Source: CAD feature listing. Evaluate the final solid. Frame: model axes, mm. A direction names the side the tool comes from. Give positions to 0.01 mm unless a question says otherwise; leave off trailing zeros. Write each loop counter-clockwise with the first axis right and the second up, starting at its lowest first coordinate (ties: lowest second). Pieces come first, ordered by that corner, then holes. Notation, with made-up numbers: M -4,37 L 5,37 A32 ccw 5,75 Z; hole C -7,-35.5 d3. An arc over 180 degrees is marked long. Return JSON: item names as keys, results as strings.
```python
from build123d import *

# Parameters (mm, degrees)
SKETCH_2_W          = 6.5
SKETCH_2_H          = 35
EXTRUDE_1_DEPTH     = 5
SKETCH_3_W          = 2.5
SKETCH_3_H          = 2
CUT_EXTRUDE_1_DEPTH = 180
SKETCH_4_W          = 6.5
SKETCH_4_H          = 19
EXTRUDE_2_DEPTH     = 26.1
SKETCH_5_W          = 6.5
SKETCH_5_H          = 15
CUT_EXTRUDE_2_DEPTH = 7


with BuildPart() as part:
    # Эскиз2 → Бобышка-Вытянуть1 (new body)
    with BuildSketch(Plane(origin=(0, 0, 0), x_dir=(1, 0, 0), z_dir=(0, 1, 0))):
        with Locations((-86.667897916, 21.515984643)):
            Rectangle(SKETCH_2_W, SKETCH_2_H)
    extrude(amount=EXTRUDE_1_DEPTH)

    # Эскиз3 → Вырез-Вытянуть1 (cut)
    with BuildSketch(Plane.XY.offset(-4.015984643)):
        with Locations((-86.667897916, 1)):
            Rectangle(SKETCH_3_W, SKETCH_3_H)
    extrude(amount=-CUT_EXTRUDE_1_DEPTH, mode=Mode.SUBTRACT)

    # Эскиз4 → Бобышка-Вытянуть2 (add)
    with BuildSketch(Plane(origin=(0, 5, 0), x_dir=(1, 0, 0), z_dir=(0, 1, 0))):
        with Locations((-86.667897916, 21.515984643)):
            Rectangle(SKETCH_4_W, SKETCH_4_H)
    extrude(amount=EXTRUDE_2_DEPTH)

    # Эскиз5 → Вырез-Вытянуть2 (cut)
    with BuildSketch(Plane(origin=(0, 31.1, 0), x_dir=(1, 0, 0), z_dir=(0, 1, 0))):
        with Locations((-86.667897916, 21.515984643)):
            Rectangle(SKETCH_5_W, SKETCH_5_H)
    extrude(amount=-CUT_EXTRUDE_2_DEPTH, mode=Mode.SUBTRACT)


solid = part.part
```
1) Set-up query: faces 1 (the face through (-87, 2, -21)), 2 (the face through (-87, 18, -31.016)), 3 (the face through (-87, 24.1, -22)). Return all of +Z, -Z, +X, -X, +Y, -Y with unobstructed straight access to the full face (end or side cutting, diameter ignored); none if empty.
Numbers:
{"face 1": "+Z, -Z, -Y", "face 2": "-Z, +X, -X, +Y", "face 3": "+X, -X, +Y"}
2) Draft query along X for faces 4 (the face through (-85.418, 1, -21)), 5 (the face through (-89.918, 12, -21)), 6 (the face through (-87, 31.1, -30)). Return one class per face: released by +X, released by -X, zero draft, split by the parting line, or undercut.
Numbers:
{"face 4": "undercut", "face 5": "released by -X", "face 6": "zero draft"}
3) Cut plane A-A, the plane y = 29.5. Return the cut outline in (x, z).
Numbers:
{"outline": "M -89.92,-31.02 L -83.42,-31.02 L -83.42,-29.02 L -89.92,-29.02 Z; M -89.92,-14.02 L -83.42,-14.02 L -83.42,-12.02 L -89.92,-12.02 Z"}
4) Cut plane C-C, the plane x = -84. Return the cut outline in (y, z).
Numbers:
{"outline": "M 0,-39.02 L 5,-39.02 L 5,-31.02 L 31.1,-31.02 L 31.1,-29.02 L 24.1,-29.02 L 24.1,-14.02 L 31.1,-14.02 L 31.1,-12.02 L 5,-12.02 L 5,-4.02 L 0,-4.02 Z"}
5) Line query: line 1 (Z direction, x = -86.75, y = 7.5); line 2 (Y direction, x = -89, z = -24); line 3 (Y direction, x = -86.5, z = -18). Output: solid intervals per line, ascending. Write a range as [from, to].
Numbers:
{"line 1": "z = [-31.02, -12.02]", "line 2": "y = [0, 24.1]", "line 3": "y = [2, 24.1]"}
6) Contact query for flat-ended pins moving along their axis: pin 1 Ø2 at (x, y) = (-86.5, 22) entering from -Z; pin 2 Ø3 at (x, z) = (-87.5, -36) entering from +Y; pin 3 Ø2 at (x, y) = (-86, 29.5) entering from +Z. Output: stop coordinate, or through.
Numbers:
{"pin 1": "stops at z = -31.02", "pin 2": "stops at y = 5", "pin 3": "stops at z = -12.02"}
7) Cut plane B-B, the plane z = -31.5. Return the cut outline in (x, y), then the cut area to 3 significant figures.
Numbers:
{"outline": "M -89.92,0 L -87.92,0 L -87.92,2 L -85.42,2 L -85.42,0 L -83.42,0 L -83.42,5 L -89.92,5 Z", "area": "27.5 mm²"}
8) Cut plane D-D, the plane x = -87.5. Return the cut outline in (y, z), then the cut area to 3 significant figures.
Numbers:
{"outline": "M 2,-39.02 L 5,-39.02 L 5,-31.02 L 31.1,-31.02 L 31.1,-29.02 L 24.1,-29.02 L 24.1,-14.02 L 31.1,-14.02 L 31.1,-12.02 L 5,-12.02 L 5,-4.02 L 2,-4.02 Z", "area": "496 mm²"}
